from build123d import *

# Parameters (mm, degrees)
SKETCH1_R           = 27
SKETCH1_R_2         = 23
BOSS_EXTRUDE1_DEPTH = 45
SKETCH1_3_R         = 1.7
BOSS_EXTRUDE2_DEPTH = 20


with BuildPart() as part:
    # Sketch1 → Boss-Extrude1 (new body)
    with BuildSketch(Plane.XY):
        Circle(SKETCH1_R)
        Circle(SKETCH1_R_2, mode=Mode.SUBTRACT)
    extrude(amount=BOSS_EXTRUDE1_DEPTH)

    # Sketch1_3 → Boss-Extrude2 (add)
    with BuildSketch(Plane.XY):
        with BuildLine():
            ThreePointArc((23, 0), (22.903113545, 2.108883576), (22.61327044, 4.2))
            Line((22.61327044, 4.2), (19, 4.2))
            ThreePointArc((19, 4.2), (14.8, 0), (19, -4.2))
            Line((19, -4.2), (22.61327044, -4.2))
            ThreePointArc((22.61327044, -4.2), (22.903113545, -2.108883576), (23, 0))
        make_face()
        with Locations((19, 0)):
            Circle(SKETCH1_3_R, mode=Mode.SUBTRACT)
        with BuildLine():
            Line((-4.2, -19), (-4.2, -22.61327044))
            ThreePointArc((-4.2, -22.61327044), (0, -23), (4.2, -22.61327044))
            Line((4.2, -22.61327044), (4.2, -19))
            ThreePointArc((4.2, -19), (0, -14.8), (-4.2, -19))
        make_face()
        with Locations((0, -19)):
            Circle(SKETCH1_3_R, mode=Mode.SUBTRACT)
        with BuildLine():
            Line((-19, 4.2), (-22.61327044, 4.2))
            ThreePointArc((-22.61327044, 4.2), (-23, 0), (-22.61327044, -4.2))
            Line((-22.61327044, -4.2), (-19, -4.2))
            ThreePointArc((-19, -4.2), (-14.8, 0), (-19, 4.2))
        make_face()
        with Locations((-19, 0)):
            Circle(SKETCH1_3_R, mode=Mode.SUBTRACT)
        with BuildLine():
            Line((-4.2, 22.61327044), (-4.2, 19))
            ThreePointArc((-4.2, 19), (0, 14.8), (4.2, 19))
            Line((4.2, 19), (4.2, 22.61327044))
            ThreePointArc((4.2, 22.61327044), (0, 23), (-4.2, 22.61327044))
        make_face()
        with Locations((0, 19)):
            Circle(SKETCH1_3_R, mode=Mode.SUBTRACT)
    extrude(amount=BOSS_EXTRUDE2_DEPTH)


solid = part.part
The model under review builds one solid part; all positions refer to its coordinate system, in mm. A direction names the side the tool comes from. Give positions to 0.01 mm unless a question says otherwise; leave off trailing zeros. Loops run counter-clockwise (first coordinate to the right, second up) from the corner with the lowest first, then second, coordinate; pieces in that order, holes last. Notation, with made-up numbers: (-9, -3) -> (12, -3) arc R7 cw to (12, 6) -> close; hole circle Ø3 at (-12.5, -1). An arc over 180 degrees is marked (long way). Answer as a JSON object with one key per item and string values. Group by question number.
Q1. Take a section at D-D (z = 29). Write out the cut boundary in (x, y).
Q2. Tool access review of faces 3 (the flat face through (1, -21, 20)), 4 (the flat face through (4.2, -21, 10)): name each direction out of +Z, -Z, +X, -X, +Y, -Y from which nothing blocks a thin tool from reaching the whole face with its end or side.
Q3. Take a section at A-A (y = 0). Write out the cut boundary in (x, z).
Q4. Draft analysis for pull direction X (two halves, no side actions). For faces 1 (the cylindrical face through (-5.85, -26.36, 22.18)), 2 (the cylindrical face through (20.57, -0.65, 9.86)), state which applies: pulls with the +X half, pulls with the -X half, needs draft (parallel to the pull), parting line crosses it, or undercut.
Q5. Wall thickness on line 1 along Y through (x, z) = (0, 11.5); line 2 along Y through (x, z) = (-19, 9.25); line 3 along X through (y, z) = (-13.5, 18.5): over which ranges is each line inside the solid? List them lowest first.
Q6. Insertion check: pin 1 (2.5 mm diameter, centred on x = -0.5, y = 18.5, fed in from +Z); pin 2 (10 mm diameter, centred on x = 2, z = 14.5, fed in from -Y); pin 3 (1.1 mm diameter, centred on x = -21, z = 12, fed in from -Y). Each pin has a flat end and moves straight along its axis. Give the tip position at first contact, or say it passes through.
Q7. Take a section at C-C (y = -10.5). Write out the cut boundary in (x, z).
Q8. Take a section at B-B (z = 4.5). Write out the cut boundary in (x, y).
Answer below:
{
 "1": {"outline": "circle Ø54 at (0, 0); hole circle Ø46 at (0, 0)"},
 "2": {"face 3": "+Z", "face 4": "+Z, -Z"},
 "3": {"outline": "(-27, 0) -> (-20.7, 0) -> (-20.7, 20) -> (-23, 20) -> (-23, 45) -> (-27, 45) -> close; (-17.3, 0) -> (-14.8, 0) -> (-14.8, 20) -> (-17.3, 20) -> close; (14.8, 0) -> (17.3, 0) -> (17.3, 20) -> (14.8, 20) -> close; (20.7, 0) -> (27, 0) -> (27, 45) -> (23, 45) -> (23, 20) -> (20.7, 20) -> close"},
 "4": {"face 1": "parting line crosses it", "face 2": "undercut"},
 "5": {"line 1": "y = -27 to -20.7, -17.3 to -14.8, 14.8 to 17.3, 20.7 to 27", "line 2": "y = -19.18 to -12.96, -4.2 to -1.7, 1.7 to 4.2, 12.96 to 19.18", "line 3": "x = -23.38 to -18.62, 18.62 to 23.38"},
 "6": {"pin 1": "stops at z = 20", "pin 2": "stops at y = -27", "pin 3": "stops at y = -17.63"},
 "7": {"outline": "(-24.87, 0) -> (-20.46, 0) -> (-20.46, 45) -> (-24.87, 45) -> close; (20.46, 0) -> (24.87, 0) -> (24.87, 45) -> (20.46, 45) -> close"},
 "8": {"outline": "circle Ø54 at (0, 0); hole (-22.61, -4.2) arc R23 ccw to (-4.2, -22.61) -> (-4.2, -19) arc R4.2 cw to (4.2, -19) -> (4.2, -22.61) arc R23 ccw to (22.61, -4.2) -> (19, -4.2) arc R4.2 cw to (19, 4.2) -> (22.61, 4.2) arc R23 ccw to (4.2, 22.61) -> (4.2, 19) arc R4.2 cw to (-4.2, 19) -> (-4.2, 22.61) arc R23 ccw to (-22.61, 4.2) -> (-19, 4.2) arc R4.2 cw to (-19, -4.2) -> close; hole circle Ø3.4 at (-19, 0); hole circle Ø3.4 at (0, -19); hole circle Ø3.4 at (0, 19); hole circle Ø3.4 at (19, 0)"}
}
